Can you work these out from the model? Positions are in its coordinate system, mm. A direction names the side the tool comes from. Give positions to 0.01 mm unless a question says otherwise; leave off trailing zeros. Write each loop counter-clockwise with the first axis right and the second up, starting at its lowest first coordinate (ties: lowest second). Pieces come first, ordered by that corner, then holes.
from build123d import *

# Parameters (mm, degrees)
F1_DEPTH = 7
F4_DEPTH = 2
F5_R     = 0.99999
F6_R     = 3


# Not quite as in the source:
# - a fillet or chamfer is up to 0.001 mm smaller than in the source, because OpenCascade refuses the exact size


with BuildPart() as f1:
    # F0 (on Front) → F1 (new body)
    with BuildSketch(Plane.XZ):
        with BuildLine():
            ThreePointArc((1.2846968546, -5.7110060848), (-2.9268599432, -3.6584002375), (0, 0))
            Line((0, 0), (50, 0))
            Line((50, 0), (50, 2))
            Line((50, 2), (0, 2))
            ThreePointArc((0, 2), (-4.8780999054, -4.0973337292), (2.1411614243, -7.5183434747))
            ThreePointArc((2.1411614243, -7.5183434747), (21.7926594555, -2.5678073417), (41.8462591278, -5.4905326207))
            ThreePointArc((41.8462591278, -5.4905326207), (43.3714151553, -5.9679500269), (44.9277769901, -6.3309460698))
            Line((44.9277769901, -6.3309460698), (45.3094672073, -4.3677057436))
            ThreePointArc((45.3094672073, -4.3677057436), (43.8976496677, -4.0384223028), (42.5141397524, -3.6053441762))
            ThreePointArc((42.5141397524, -3.6053441762), (21.6906488053, -0.5704105791), (1.2846968546, -5.7110060848))
        make_face()
    extrude(amount=F1_DEPTH)

    # F3 (on face) → F4 (cut)
    with BuildSketch(Plane.XY.offset(2)):
        Polygon((0, -2), (941.9215958638, -2), (50, 0), (0, 0), align=None)
        Polygon((941.9215958638, -5), (0, -5), (0, -7), (0.1395036115, -8.5481454325), (941.9215958638, -6.9726880672), align=None)
    extrude(amount=-F4_DEPTH, mode=Mode.SUBTRACT)

    # F5 (radius 1 in the source; OpenCascade refuses exactly that, so slightly less here)
    f5_edges = [f1.edges().sort_by_distance(p)[0] for p in [
        (0, 0, 1),
        (0, -5, 1),
        (50, -5, 1),
        (50, -2, 1),
        (0, -7, 1),
        (0, -2, 1),
    ]]
    fillet(f5_edges, radius=F5_R)

    # F6
    f6_edges = [f1.edges().sort_by_distance(p)[0] for p in [
        (45.118622, -7, -5.349326),
        (45.118622, 0, -5.349326),
    ]]
    fillet(f6_edges, radius=F6_R)


solid = f1.part
(1) Imagine slicing it at B-B, the plane z = -3. Write out the boundary of the cut face in (x, y), plus the area to 3 significant figures.
Returned:
outline: (-5, -7) - (-3, -7) - (-3, 0) - (-5, 0) - close; (8.19, -7) - (17.25, -7) - (17.25, 0) - (8.19, 0) - close; (31.65, -7) - (40.7, -7) - (40.7, 0) - (31.65, 0) - close
area: 141 mm2
(2) Imagine slicing it at A-A, the plane x = 32. Write out the boundary of the cut face in (y, z).
Returned:
outline: (-7, -3.05) - (0, -3.05) - (0, -1.03) - (-7, -1.03) - close; (-5, 0) - (-2, 0) - (-2, 2) - (-5, 2) - close
(3) If we mould it in two halves opening along X, with no side actions, what happens to faces 1 (the face through (25, -3, 0)), 2 (the face through (-2.91, -3.45, -3.73)), 3 (the face through (0.285, -1.699, 0.986))? For each: +X half, -X half, draft (parallel to the pull), parting line (faces both ways), or undercut.
Returned:
face 1: draft
face 2: undercut
face 3: +X half
(4) Imagine slicing it at D-D, the plane x = 12.5. Write out the boundary of the cut face in (y, z).
Returned:
outline: (-7, -3.89) - (0, -3.89) - (0, -1.84) - (-7, -1.84) - close; (-5, 0) - (-2, 0) - (-2, 2) - (-5, 2) - close
(5) If I drill on L1, parallel to Z at x = 0, y = -5; L2, parallel to X at y = -4, z = 0.5; L3, parallel to Y at x = 3.5, z = 0.5, over which ranges is the centre line in solid material (lowest first)?
Returned:
L1: z = -8 to -6, 0 to 2
L2: x = -3.57 to 50
L3: y = -5 to -2
(6) Will these pins go through, and if not, where does the flat tip stop? P1, Ø1.5, axis at x = 24.5, y = -2.5, coming from the -Z side; P2, Ø1.6, axis at x = 30.5, z = 0.5, coming from the -Y side; P3, Ø1, axis at x = 24.5, z = 1, coming from the +Y side.
Returned:
P1: stops at z = -2.51
P2: stops at y = -5
P3: stops at y = -2
(7) Imagine slicing it at C-C, the plane y = -5.5. Write out the boundary of the cut face in (x, z).
Returned:
outline: (0, 0) - (0.13, 0) - (0.13, 2) - (0, 2) arc R5 ccw (long way) to (2.14, -7.52) arc R52.09 cw to (41.85, -5.49) arc R21.53 ccw to (44.53, -6.25) - (44.92, -4.29) arc R19.53 cw to (42.51, -3.61) arc R54.09 ccw to (1.28, -5.71) arc R3 cw (long way) to start
(8) For faces 4 (the face through (43.607, -3.451, -3.957)), 5 (the face through (-0.285, -6.699, 0.899)), 6 (the face through (-0.285, -0.301, 0.899)), which set-ups out of +Z, -Z, +X, -X, +Y, -Y let a thin tool reach every point of the face, with its end or its side?
Returned:
face 4: +X, +Y, -Y
face 5: +Z, +X, -Y
face 6: +Z, +X, +Y
